from build123d import *

# Parameters (mm, degrees)
CYLINDER005_R     = 1.5
CYLINDER005_DEPTH = 10
ARRAY007_COUNT    = 3
TUBE014_R         = 15
TUBE014_R_2       = 2.75
TUBE014_DEPTH     = 2.5
BOX001_W          = 10
BOX001_H          = 1.5
BOX001_DEPTH      = 8.2
BOX_W             = 4.5
BOX_H             = 4.5
BOX_DEPTH         = 32.5
CYLINDER026_R     = 1.2
CYLINDER026_DEPTH = 18.5
CYLINDER027_R     = 1.2
CYLINDER027_DEPTH = 18.5
BOX021_W          = 4.5
BOX021_H          = 4.5
BOX021_DEPTH      = 36


with BuildPart() as pistonconnectorscrewcutters:
    # Cylinder005 → Cylinder005 (new body)
    with BuildSketch(Plane(origin=(6.5, 0, 110), x_dir=(1, 0, 0), z_dir=(0, 0, 1))):
        Circle(CYLINDER005_R)
    extrude(amount=CYLINDER005_DEPTH)

    # Array007: PistonConnectorScrewCutters ×3 about axis
    array007_axis = Axis((0, 0, 0), (0, 0, 1))


with BuildPart() as pistonconnectorscrewcutters_1:
    add(pistonconnectorscrewcutters.part)
    for i in range(1, ARRAY007_COUNT):
        add(pistonconnectorscrewcutters.part.rotate(array007_axis, i * 360 / ARRAY007_COUNT))


with BuildPart() as obj1:
    # Tube014 → Tube014 (new body)
    with BuildSketch(Plane.XY.offset(115)):
        Circle(TUBE014_R)
        Circle(TUBE014_R_2, mode=Mode.SUBTRACT)
    extrude(amount=TUBE014_DEPTH)


with BuildPart() as obj2:
    # Box001 → Box001 (new body)
    with BuildSketch(Plane(origin=(7, -0.75, 139.5), x_dir=(1, 0, 0), z_dir=(0, 0, 1))):
        with Locations((5, 0.75)):
            Rectangle(BOX001_W, BOX001_H)
    extrude(amount=BOX001_DEPTH)


with BuildPart() as obj3:
    # Box → Box (new body)
    with BuildSketch(Plane(origin=(10, -2.25, 117.5), x_dir=(1, 0, 0), z_dir=(0, 0, 1))):
        with Locations((2.25, 2.25)):
            Rectangle(BOX_W, BOX_H)
    extrude(amount=BOX_DEPTH)

    # Cut001: cut obj2
    add(obj2.part, mode=Mode.SUBTRACT)

    # Fusion004: union obj1
    add(obj1.part)

    # Cut033: cut PistonConnectorScrewCutters
    add(pistonconnectorscrewcutters_1.part, mode=Mode.SUBTRACT)


with BuildPart() as safetybuttonshookscrewcutter:
    # Cylinder026 → Cylinder026 (new body)
    with BuildSketch(Plane(origin=(-28.5, 0, 150.5), x_dir=(0, 0, -1), z_dir=(1, 0, 0))):
        Circle(CYLINDER026_R)
    extrude(amount=CYLINDER026_DEPTH)


with BuildPart() as obj4:
    # Cylinder027 → Cylinder027 (new body)
    with BuildSketch(Plane(origin=(-28.5, 0, 145.5), x_dir=(0, 0, -1), z_dir=(1, 0, 0))):
        Circle(CYLINDER027_R)
    extrude(amount=CYLINDER027_DEPTH)

    # Fusion013: union SafetyButtonsHookScrewCutter
    add(safetybuttonshookscrewcutter.part)


with BuildPart() as pistonhooks:
    # Box021 → Box021 (new body)
    with BuildSketch(Plane(origin=(-14.5, -2.25, 117.5), x_dir=(1, 0, 0), z_dir=(0, 0, 1))):
        with Locations((2.25, 2.25)):
            Rectangle(BOX021_W, BOX021_H)
    extrude(amount=BOX021_DEPTH)

    # Cut050: cut obj4
    add(obj4.part, mode=Mode.SUBTRACT)

    # Fusion014: union obj3
    add(obj3.part)


solid = pistonhooks.part
Design review of the part built by this model. Coordinates are the model's own, in mm. A direction names the side the tool comes from. Round coordinates to 2 decimals unless told otherwise and drop trailing zeros. Write each loop counter-clockwise with the first axis right and the second up, starting at its lowest first coordinate (ties: lowest second). Pieces come first, ordered by that corner, then holes. Notation, with made-up numbers: (-4.5, 51) -> (3.5, 51) arc R23 ccw to (3.5, 90) -> close; hole circle Ø4 at (85, 66). An arc over 180 degrees is marked (long way). One line per question, with ' | ' between items.
(1) Machinability: for faces 1 (the flat face through (14.5, 0, 134)), 2 (the flat face through (12, 0, 139.5)), 3 (the flat face through (-12, -2.25, 135)), which of the approach directions +Z, -Z, +X, -X, +Y, -Y give a long, thin tool a straight path to every point of the face, cutting with its end or side? Answer none if there is none.
Result sheet:
face 1: +Z, +X, +Y, -Y | face 2: +X | face 3: +Z, +X, -X, -Y
(2) Take a section at C-C, the plane z = 150.5. State the section outline as (x, y) points, and give its area (3 significant figures).
Result sheet:
outline: (-14.5, -2.25) -> (-10, -2.25) -> (-10, -1.2) -> (-14.5, -1.2) -> close; (-14.5, 1.2) -> (-10, 1.2) -> (-10, 2.25) -> (-14.5, 2.25) -> close | area: 9.45 mm2
(3) Draft analysis for pull direction Y (two halves, no side actions). For faces 4 (the flat face through (12, 0.75, 144)), 5 (the cylindrical face through (-14.985, 0.66, 116.232)), 6 (the flat face through (3, 0, 117.5)), state which applies: released by +Y, released by -Y, zero draft, split by the parting line, or undercut.
Result sheet:
face 4: undercut | face 5: split by the parting line | face 6: zero draft
(4) Take a section at A-A, the plane z = 143. State the section outline as (x, y) points, and give its area (4 significant figures).
Result sheet:
outline: (-14.5, -2.25) -> (-10, -2.25) -> (-10, 2.25) -> (-14.5, 2.25) -> close; (10, -2.25) -> (14.5, -2.25) -> (14.5, -0.75) -> (10, -0.75) -> close; (10, 0.75) -> (14.5, 0.75) -> (14.5, 2.25) -> (10, 2.25) -> close | area: 33.75 mm2
(5) Wall thickness on line 1 (Y direction, x = -13.1, z = 150.5); line 2 (X direction, y = 1.5, z = 134); line 3 (Y direction, x = -3.25, z = 116.8): over which ranges is each line inside the solid? List them lowest first. Write a range as [from, to].
Result sheet:
line 1: [-2.25, -1.2], [1.2, 2.25] | line 2: [-14.5, -10], [10, 14.5] | line 3: [-14.64, -7.13], [-4.13, 4.13], [7.13, 14.64]
(6) Take a section at B-B, the plane x = 0. State the section outline as (y, z) points.
Result sheet:
outline: (-15, 115) -> (-2.75, 115) -> (-2.75, 117.5) -> (-15, 117.5) -> close; (2.75, 115) -> (15, 115) -> (15, 117.5) -> (2.75, 117.5) -> close
(7) Insertion check: P1, Ø2, axis at x = 12, z = 144, coming from the -Y side; P2, Ø12, axis at y = 4.5, z = 149, coming from the +X side; P3, Ø12, axis at y = -2, z = 149.5, coming from the -X side. Each pin has a flat end and moves straight along its axis. Give the tip position at first contact, or say it passes through.
Result sheet:
P1: y = -2.25 | P2: x = 14.5 | P3: x = -14.5
(8) Take a section at D-D, the plane y = 0. State how many separate pieces and enclosed holes the cut face has, and give its area (4 significant figures).
Result sheet:
separate pieces: 6 | enclosed holes: 0 | area: 303.5 mm2
